```python
from build123d import *

# Parameters (mm, degrees)
SKETCH1_R               = 6
SKETCH1_R_2             = 2.5
BOSS_EXTRUDE1_DEPTH     = 9
SKETCH2_R               = 1.5
BOSS_EXTRUDE2_DEPTH     = 6
CUT_EXTRUDE2_DEPTH      = 22.863211109
CUT_EXTRUDE2_DEPTH_BACK = 22.863211109
SKETCH5_W               = 8.5
SKETCH5_H               = 12


with BuildPart() as part:
    # Sketch1 → Boss-Extrude1 (new, symmetric)
    with BuildSketch(Plane.XY):
        Circle(SKETCH1_R)
        Circle(SKETCH1_R_2, mode=Mode.SUBTRACT)
    extrude(amount=BOSS_EXTRUDE1_DEPTH, both=True)

    # Sketch2 → Boss-Extrude2 (add, symmetric)
    with BuildSketch(Plane(origin=(0, 0, 0), x_dir=(1, 0, 0), z_dir=(0, 1, 0))):
        with BuildLine():
            Line((0, 9), (16, 9))
            ThreePointArc((16, 9), (18.121320344, 8.121320344), (19, 6))
            Line((19, 6), (19, -6))
            ThreePointArc((19, -6), (18.121320344, -8.121320344), (16, -9))
            Line((16, -9), (0, -9))
            Line((0, -9), (0, 9))
        make_face()
        with Locations(Location((16, 6, 0), (0, 0, 270))):
            Circle(SKETCH2_R, mode=Mode.SUBTRACT)
        with Locations(Location((16, -6, 0), (0, 0, 270))):
            Circle(SKETCH2_R, mode=Mode.SUBTRACT)
    extrude(amount=BOSS_EXTRUDE2_DEPTH, both=True)

    # Sketch3 → Cut-Revolve1 (revolve, cut)
    with BuildSketch(Plane(origin=(0, 0, 0), x_dir=(1, 0, 0), z_dir=(0, 1, 0)), mode=Mode.PRIVATE) as cut_revolve1_sk:
        Polygon((2.5, 8), (2.5, 9), (0, 9), (0, -9), (2.5, -9), (2.5, -8), (3, -8), (3, -6), (4.5, -6), (4.5, 6), (3, 6), (3, 8), align=None)
    revolve(cut_revolve1_sk.sketch.rotate(Axis((0, 0, -12.234149704), (0, 0, 1)), 180), axis=Axis((0, 0, -12.234149704), (0, 0, 1)), mode=Mode.SUBTRACT)

    # Sketch5 → Cut-Extrude2 (cut, two sides: drawn at the far end of the back side and taken through both)
    with BuildSketch(Plane(origin=(0, 0, 0), x_dir=(1, 0, 0), z_dir=(0, 1, 0)).offset(-CUT_EXTRUDE2_DEPTH_BACK)):
        with Locations((-1.75, 0)):
            Rectangle(SKETCH5_W, SKETCH5_H)
    extrude(amount=CUT_EXTRUDE2_DEPTH + CUT_EXTRUDE2_DEPTH_BACK, mode=Mode.SUBTRACT)


solid = part.part
```
Could you check a few things on this model? Use its own coordinates, in mm. A direction names the side the tool comes from. Round coordinates to 2 decimals unless told otherwise and drop trailing zeros. Loops run counter-clockwise (first coordinate to the right, second up) from the corner with the lowest first, then second, coordinate; pieces in that order, holes last.
Q1. On a 3-axis mill with a long thin cutter (end or side, diameter ignored), from which of +Z, -Z, +X, -X, +Y, -Y can I reach the whole of each face in a straight line? I mean faces 1 (the flat face through (2.5, -5, 0)), 2 (the cylindrical face through (-2.86, -0.9, -7.01)), 3 (the flat face through (19, 0, 0)), 4 (the flat face through (-3.2, -0.1, 6)), 5 (the cylindrical face through (18.14, 0.08, 8.1)). Say none if no direction works.
Q2. I want a section at D-D (y = -4.5). Write out the boundary of the cut face in (x, z), and give its area (3 significant figures).
Q3. I want a section at A-A (y = 0). Write out the boundary of the cut face in (x, z), and give its area (3 significant figures).
Q4. I want a section at C-C (x = 2). Write out the boundary of the cut face in (y, z).
Q5. Thinking about a two-plate mould opening in Y: for faces 6 (the cylindrical face through (18.1, 0.08, -8.14)), 7 (the flat face through (-2, -2, 8)), 8 (the flat face through (10, -6, 0)), 9 (the flat face through (2, -2, -8)), which applies, pulls with the +Y half, pulls with the -Y half, needs draft (parallel to the pull), parting line crosses it, or undercut?
Q6. I want a section at B-B (z = 1.25). Write out the boundary of the cut face in (x, y), and give its area (3 significant figures).
Q7. Please list where these lines run through material, in increasing order: L1, parallel to Y at x = 0, z = -6.75; L2, parallel to Z at x = -4.25, y = -2.75; L3, parallel to Z at x = 2.5, y = 0.5.
Q8. For P1, Ø0.7, axis at y = 5, z = 2, coming from the -X side, with a flat end and sliding along its axis, tell me the tip position at first contact or that it passes through.
Answer below:
1. face 1: -X, +Y, -Y
1. face 2: none
1. face 3: +Z, -Z, +X, +Y, -Y
1. face 4: -X
1. face 5: +Z, +X, +Y, -Y
2. outline: (-3.97, -9) - (16, -9) arc R3 ccw to (19, -6) - (19, 6) arc R3 ccw to (16, 9) - (-3.97, 9) - (-3.97, 6) - (2.5, 6) - (2.5, -6) - (-3.97, -6) - close; hole circle Ø3 at (16, -6); hole circle Ø3 at (16, 6)
2. area: 318 mm2
3. outline: (-6, -9) - (-2.5, -9) - (-2.5, -8) - (-3, -8) - (-3, -6) - (-6, -6) - close; (-6, 6) - (-3, 6) - (-3, 8) - (-2.5, 8) - (-2.5, 9) - (-6, 9) - close; (2.5, -9) - (16, -9) arc R3 ccw to (19, -6) - (19, 6) arc R3 ccw to (16, 9) - (2.5, 9) - (2.5, 8) - (3, 8) - (3, 6) - (4.5, 6) - (4.5, -6) - (3, -6) - (3, -8) - (2.5, -8) - close; hole circle Ø3 at (16, -6); hole circle Ø3 at (16, 6)
3. area: 272 mm2
4. outline: (-6, -9) - (-1.5, -9) - (-1.5, -8) - (-2.24, -8) - (-2.24, -6) - (-6, -6) - close; (-6, 6) - (-2.24, 6) - (-2.24, 8) - (-1.5, 8) - (-1.5, 9) - (-6, 9) - close; (1.5, -9) - (6, -9) - (6, -6) - (2.24, -6) - (2.24, -8) - (1.5, -8) - close; (1.5, 8) - (2.24, 8) - (2.24, 6) - (6, 6) - (6, 9) - (1.5, 9) - close
5. face 6: needs draft
5. face 7: undercut
5. face 8: pulls with the -Y half
5. face 9: undercut
6. outline: (2.5, -6) - (19, -6) - (19, 6) - (2.5, 6) - (2.5, 3.74) arc R4.5 cw to (2.5, -3.74) - close
6. area: 187 mm2
7. L1: y = -6 to -3, 3 to 6
7. L2: z = -9 to -6, 6 to 9
7. L3: z = -9 to -8, 8 to 9
8. P1: stops at x = 2.5
